```python
from build123d import *

# Parameters (mm, degrees)
SKETCH_1_W           = 36
SKETCH_1_H           = 219
EXTRUDE_1_DEPTH      = 37
SKETCH_2_W           = 80.767995678
SKETCH_2_H           = 159
CUT_EXTRUDE_1_DEPTH  = 117.975424769
CUT_EXTRUDE_START    = 10
SKETCH_9_W           = 26
SKETCH_9_H           = 219
CUT_EXTRUDE_7_DEPTH  = 17
SKETCH_10_W          = 12
SKETCH_10_H          = 236
CUT_EXTRUDE_8_DEPTH  = 17
CUT_EXTRUDE_START_2  = 37
SKETCH_11_R          = 3.5
CUT_EXTRUDE_11_DEPTH = 17
SKETCH_25_R          = 15
EXTRUDE_3_DEPTH      = 40


with BuildPart() as part:
    # 스케치1 → 보스-돌출1 (new body)
    with BuildSketch(Plane.XY):
        Rectangle(SKETCH_1_W, SKETCH_1_H)
    extrude(amount=EXTRUDE_1_DEPTH)

    # 스케치2 → 컷-돌출1 (cut, through all)
    with BuildSketch(Plane.XY):
        with Locations((32.383997839, -3)):
            Rectangle(SKETCH_2_W, SKETCH_2_H)
    extrude(amount=CUT_EXTRUDE_1_DEPTH, mode=Mode.SUBTRACT)

    # 스케치9 → 컷-돌출7 (cut)
    with BuildSketch(Plane.XY.offset(CUT_EXTRUDE_START)):
        with Locations((5, 0)):
            Rectangle(SKETCH_9_W, SKETCH_9_H)
    extrude(amount=CUT_EXTRUDE_7_DEPTH, mode=Mode.SUBTRACT)

    # 스케치10 → 컷-돌출8 (cut)
    with BuildSketch(Plane.XY):
        with Locations((12, 8.5)):
            Rectangle(SKETCH_10_W, SKETCH_10_H)
    extrude(amount=CUT_EXTRUDE_8_DEPTH, mode=Mode.SUBTRACT)

    # 스케치11 → 컷-돌출11 (cut)
    with BuildSketch(Plane.XY.offset(CUT_EXTRUDE_START_2)):
        with Locations((3.878169626, 88)):
            Circle(SKETCH_11_R)
        with Locations((3.878169626, -92)):
            Circle(SKETCH_11_R)
    extrude(amount=-CUT_EXTRUDE_11_DEPTH, mode=Mode.SUBTRACT)

    # 스케치25 → 보스-돌출3 (add)
    with BuildSketch(Plane.ZY.offset(18)):
        with Locations(Location((18.5, 0, 0), (0, 0, 180))):
            Circle(SKETCH_25_R)
    extrude(amount=EXTRUDE_3_DEPTH)


solid = part.part
```
Here's how the part is built. I have some questions about the finished solid (model axes, mm). A direction names the side the tool comes from. Give positions to 0.01 mm unless a question says otherwise; leave off trailing zeros. Order: outer loops, then holes, each group sorted by start corner. A loop starts at its lowest first (then second) coordinate and runs counter-clockwise, first axis right, second up. Notation, with made-up numbers: (9.5, 22.5) -> (27.5, 22.5) arc R23 cw to (27.5, 37.5) -> close; hole circle Ø3 at (28.5, 86.25). An arc over 180 degrees is marked (long way). Use CSV: the item, a comma, the result in double quotes. Start each with the question number.
Item 1: Thinking about a two-plate mould opening in Y: for faces 1 (the flat face through (-58, 0, 19)), 2 (the flat face through (-1, 76.5, 5)), 3 (the flat face through (-8.3, 109.5, 18.2)), which applies, pulls with the +Y half, pulls with the -Y half, needs draft (parallel to the pull), parting line crosses it, or undercut?
Item 2: Suppose I cut it at A-A (x = -2). List the corners of the cut face in (y, z) for me, and give its area (3 significant figures).
Item 3: I'm going to push flat-ended pins straight in: P1, Ø8, axis at x = -2, z = 16.5, coming from the -Y side; P2, Ø11, axis at y = -33.5, z = 17.5, coming from the -X side; P3, Ø2, axis at x = -28, y = -4, coming from the -Z side; P4, Ø12, axis at x = -23, y = -85.5, coming from the +Z side. Where does each tip first touch, or does it pass through?
Item 4: Suppose I cut it at D-D (z = 31.5). List the corners of the cut face in (x, y) for me, and give its area (3 significant figures).
Item 5: Suppose I cut it at C-C (y = 88). List the corners of the cut face in (x, z) for me.
Item 6: If I drill on probe 1 along Y at (x, z) = (1, 32.5); probe 2 along Y at (x, z) = (-2, 3); probe 3 along Z at (x, y) = (9, 78.5), over which ranges is the centre line in solid material (lowest first)? Write a range as [from, to].
Item 7: Suppose I cut it at B-B (z = 18.5). List the corners of the cut face in (x, y) for me.
Item 8: On a 3-axis mill with a long thin cutter (end or side, diameter ignored), from which of +Z, -Z, +X, -X, +Y, -Y can I reach the whole of each face in a straight line? I mean faces 4 (the flat face through (-1, -82.5, 5)), 5 (the flat face through (5, -96, 27)), 6 (the cylindrical face through (3.119, 84.583, 32.07)), 7 (the flat face through (6, -96, 5)). Say none if no direction works.
Answer block:
1,face 1,"needs draft"
1,face 2,"undercut"
1,face 3,"pulls with the +Y half"
2,outline,"(-109.5, 0) -> (-82.5, 0) -> (-82.5, 10) -> (-109.5, 10) -> close; (-109.5, 27) -> (-82.5, 27) -> (-82.5, 37) -> (-109.5, 37) -> close; (76.5, 0) -> (109.5, 0) -> (109.5, 10) -> (76.5, 10) -> close; (76.5, 27) -> (109.5, 27) -> (109.5, 37) -> (76.5, 37) -> close"
2,area,"1,200 mm^2"
3,P1,"passes through"
3,P2,"stops at x = -18"
3,P3,"stops at z = 3.8"
3,P4,"stops at z = 37"
4,outline,"(-58, -7.48) -> (-18, -7.48) -> (-18, -109.5) -> (18, -109.5) -> (18, -82.5) -> (-8, -82.5) -> (-8, 76.5) -> (18, 76.5) -> (18, 109.5) -> (-18, 109.5) -> (-18, 7.48) -> (-58, 7.48) -> close; hole circle Ø7 at (3.88, -92); hole circle Ø7 at (3.88, 88)"
4,area,"4,270 mm^2"
5,outline,"(-18, 0) -> (6, 0) -> (6, 10) -> (-8, 10) -> (-8, 27) -> (0.38, 27) -> (0.38, 37) -> (-18, 37) -> close; (7.38, 27) -> (18, 27) -> (18, 37) -> (7.38, 37) -> close"
6,probe 1,"y = [-109.5, -93.99], [-90.01, -82.5], [76.5, 86.01], [89.99, 109.5]"
6,probe 2,"y = [-109.5, -82.5], [76.5, 109.5]"
6,probe 3,"z = [27, 37]"
7,outline,"(-58, -15) -> (-18, -15) -> (-18, -109.5) -> (-8, -109.5) -> (-8, 109.5) -> (-18, 109.5) -> (-18, 15) -> (-58, 15) -> close"
8,face 4,"+Z, -Z, +X"
8,face 5,"+X, +Y, -Y"
8,face 6,"+Z"
8,face 7,"-Z, +X, +Y, -Y"
